Build history of the part. All positions in model axes, mm. Face numbers are marked on the shaded views. A direction names the side the tool comes from. Round coordinates to 2 decimals unless told otherwise and drop trailing zeros. Loops run counter-clockwise (first coordinate to the right, second up) from the corner with the lowest first, then second, coordinate; pieces in that order, holes last. Notation, with made-up numbers: (67.5, -16) - (96.5, -16) arc R7 cw to (96.5, -11) - close; hole circle Ø11 at (0.25, -28.75). An arc over 180 degrees is marked (long way). Use one line per item in the form item = value. Start each with the question number.
Q1. Pin check, flat tips, straight feed: pin 1 (1 mm diameter, centred on x = -4.5, y = 18, fed in from -Z); pin 2 (2.5 mm diameter, centred on x = 3, z = 28, fed in from +Y); pin 3 (5 mm diameter, centred on x = 30, z = 9.5, fed in from +Y). Stop position of each tip, or through.
Q2. Saw through at B-B (z = -6.5). Give the cut face in (x, y).
Q3. Saw through at C-C (x = -12.5). Give the cut face in (y, z).
Q4. Saw through at A-A (y = 58.5). Give the cut face in (x, z), then the cut area to 3 significant figures.
Q5. Saw through at D-D (x = 30). Give the cut face in (y, z).
Q6. Drill centre lines: line 1 (Y direction, x = -15.5, z = 0); line 2 (X direction, y = 179, z = -21); line 3 (Y direction, x = 15, z = 0). Where is each one in solid material? Low to high.
Q7. 3-axis set-ups, long thin cutter, end or side, ignore diameter. For the marked faces 1, 2 and 3: which of +Z, -Z, +X, -X, +Y, -Y reach the whole face in a straight line?
Q8. Mould opens along Z. For the marked faces 4, 5, 6 and 7 say: released by +Z, released by -Z, zero draft, split by the parting line, or undercut.
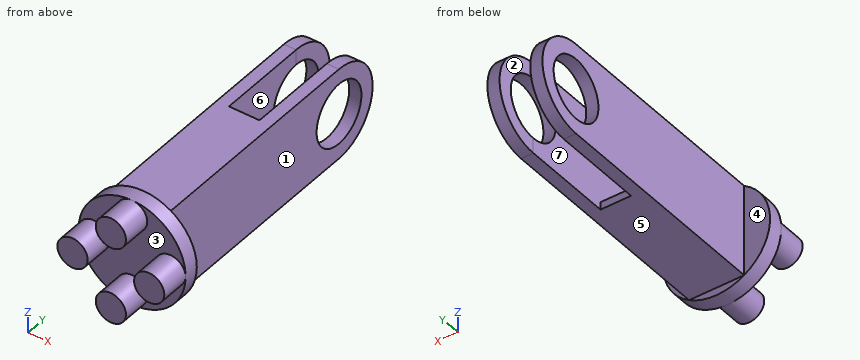
```python
from build123d import *

# Parameters (mm, degrees)
SKETCH1_R            = 35
BOSS_EXTRUDE1_DEPTH  = 10
SKETCH3_R            = 9.9
BOSS_EXTRUDE2_DEPTH  = 19
SKETCH4_W            = 36.055512754
SKETCH4_H            = 60
BOSS_EXTRUDE8_DEPTH  = 150
SKETCH11_W           = 20
SKETCH11_H           = 60
CUT_EXTRUDE2_DEPTH   = 60
SKETCH12_W           = 20
SKETCH12_H           = 50
CUT_EXTRUDE3_DEPTH   = 90
SKETCH13_R           = 30
BOSS_EXTRUDE9_DEPTH  = 8
SKETCH14_R           = 30
BOSS_EXTRUDE10_DEPTH = 8
SKETCH15_R           = 20
CUT_EXTRUDE4_DEPTH   = 97


with BuildPart() as part:
    # Sketch1 → Boss-Extrude1 (new body)
    with BuildSketch(Plane(origin=(0, 0, 0), x_dir=(1, 0, 0), z_dir=(0, 1, 0))):
        Circle(SKETCH1_R)
    extrude(amount=BOSS_EXTRUDE1_DEPTH)

    # Sketch3 → Boss-Extrude2 (add)
    with BuildSketch(Plane.XZ):
        with Locations((25.1, 0)):
            Circle(SKETCH3_R)
        with Locations((0, -25.1)):
            Circle(SKETCH3_R)
        with Locations((-25.1, 0)):
            Circle(SKETCH3_R)
        with Locations((0, 25.1)):
            Circle(SKETCH3_R)
    extrude(amount=BOSS_EXTRUDE2_DEPTH)

    # Sketch4 → Boss-Extrude8 (add)
    with BuildSketch(Plane(origin=(0, 10, 0), x_dir=(1, 0, 0), z_dir=(0, 1, 0))):
        Rectangle(SKETCH4_W, SKETCH4_H)
    extrude(amount=BOSS_EXTRUDE8_DEPTH)

    # Sketch11 → Cut-Extrude2 (cut)
    with BuildSketch(Plane(origin=(0, 160, 0), x_dir=(1, 0, 0), z_dir=(0, 1, 0))):
        Rectangle(SKETCH11_W, SKETCH11_H)
    extrude(amount=-CUT_EXTRUDE2_DEPTH, mode=Mode.SUBTRACT)

    # Sketch12 → Cut-Extrude3 (cut)
    with BuildSketch(Plane(origin=(0, 100, 0), x_dir=(1, 0, 0), z_dir=(0, 1, 0))):
        Rectangle(SKETCH12_W, SKETCH12_H)
    extrude(amount=-CUT_EXTRUDE3_DEPTH, mode=Mode.SUBTRACT)

    # Sketch13 → Boss-Extrude9 (add)
    with BuildSketch(Plane.ZY.offset(18.027756377)):
        with Locations((0, 160)):
            Circle(SKETCH13_R)
    extrude(amount=-BOSS_EXTRUDE9_DEPTH)

    # Sketch14 → Boss-Extrude10 (add)
    with BuildSketch(Plane(origin=(18.027756377, 0, 0), x_dir=(0, 0, -1), z_dir=(1, 0, 0))):
        with Locations((0, 160)):
            Circle(SKETCH14_R)
    extrude(amount=-BOSS_EXTRUDE10_DEPTH)

    # Sketch15 → Cut-Extrude4 (cut)
    with BuildSketch(Plane(origin=(18.027756377, 0, 0), x_dir=(0, 0, -1), z_dir=(1, 0, 0))):
        with Locations((0, 160)):
            Circle(SKETCH15_R)
    extrude(amount=-CUT_EXTRUDE4_DEPTH, mode=Mode.SUBTRACT)


solid = part.part
```
Report:
q1.pin_1 = -30
q1.pin_2 = 100
q1.pin_3 = 10
q2.outline = (-34.39, 0) - (-32.57, 0) - (-32.57, -19) - (-17.63, -19) - (-17.63, 0) - (17.63, 0) - (17.63, -19) - (32.57, -19) - (32.57, 0) - (34.39, 0) - (34.39, 10) - (18.03, 10) - (18.03, 141.09) - (10, 141.09) - (10, 10) - (-10, 10) - (-10, 141.09) - (-18.03, 141.09) - (-18.03, 10) - (-34.39, 10) - close; (-18.03, 178.91) - (-10.03, 178.91) - (-10.03, 189.29) - (-18.03, 189.29) - close; (10.03, 178.91) - (18.03, 178.91) - (18.03, 189.29) - (10.03, 189.29) - close
q3.outline = (0, -32.69) - (10, -32.69) - (10, -30) - (160, -30) arc R30 ccw to (160, 30) - (10, 30) - (10, 32.69) - (0, 32.69) - close; hole circle Ø40 at (160, 0)
q4.outline = (-18.03, -30) - (18.03, -30) - (18.03, 30) - (-18.03, 30) - close; hole (-10, -25) - (10, -25) - (10, 25) - (-10, 25) - close
q4.area = 1,160 mm²
q5.outline = (-19, -8.6) - (0, -8.6) - (0, -18.03) - (10, -18.03) - (10, 18.03) - (0, 18.03) - (0, 8.6) - (-19, 8.6) - close
q6.line_1 = -19 to 140, 180 to 190
q6.line_2 = -18.03 to -10.03, 10.03 to 18.03
q6.line_3 = 0 to 140, 180 to 190
q7.face_1 = +Z, -Z, +X, +Y
q7.face_2 = +Z, -Z, +Y
q7.face_3 = -Y
q8.face_4 = zero draft
q8.face_5 = released by -Z
q8.face_6 = undercut
q8.face_7 = undercut
